Geometry: final body of the model. Coordinates: model frame, mm. A direction names the side the tool comes from. Coordinates: 2 decimals unless noted, no trailing zeros. Loops run counter-clockwise (first coordinate to the right, second up) from the corner with the lowest first, then second, coordinate; pieces in that order, holes last. Notation, with made-up numbers: (17.5, 7.5) -> (36.5, 7.5) arc R29 ccw to (36.5, 38.5) -> close; hole circle Ø2 at (89, 39). An arc over 180 degrees is marked (long way). One line per item, written item: value. Start each with the question number.
Item 1: Ray query, probe 1 along X at (y, z) = (60, 21); probe 2 along Y at (x, z) = (37.5, 12); probe 3 along Z at (x, y) = (37, -56.5). Return the intervals inside material, ascending. Write a range as from..to.
Item 2: Set-up query: faces 1 (the flat face through (1, 60, 30)), 2 (the cylindrical face through (39.81, 59.04, 14.79)), 3 (the flat face through (1, -41, 25)). Return all of +Z, -Z, +X, -X, +Y, -Y with unobstructed straight access to the full face (end or side cutting, diameter ignored); none if empty.
Item 3: Contact query for flat-ended pins moving along their axis: pin 1 Ø4 at (x, y) = (-37.5, 60) entering from +Z; pin 2 Ø2 at (x, y) = (26.5, 43.5) entering from -Z; pin 3 Ø4 at (x, y) = (22.5, -21) entering from +Z; pin 4 Ø3 at (x, y) = (-14, 59.5) entering from +Z. Output: stop coordinate, or through.
Item 4: Section query D-D on z = 32.5. Return loops of the section in (x, y).
Item 5: Section query A-A on y = -60. Return loops of the section in (x, z).
Item 6: Mould query, pull axis X, two halves, no side actions, for faces 4 (the flat face through (42.5, -1, 15)), 5 (the cylindrical face through (-36, -58, 12)), 6 (the flat face through (1, -7, 33)). Classes: +X half, -X half, draft (parallel to the pull), parting line (faces both ways), or undercut.
Item 7: Section query C-C on x = -25. Return loops of the section in (y, z).
Item 8: Section query B-B on x = -37.5. Return loops of the section in (y, z), then the cut area to 3 significant figures.
from build123d import *

# Parameters (mm, degrees)
SCHIZZO1_W                   = 85
SCHIZZO1_H                   = 130
SCHIZZO1_R                   = 2.5
ESTRUSIONE_ESTRUSIONE1_DEPTH = 40
TAGLIO_ESTRUSIONE1_DEPTH     = 115.236596588


with BuildPart() as part:
    # Schizzo1 → Estrusione-Estrusione1 (new body)
    with BuildSketch(Plane.XY):
        Rectangle(SCHIZZO1_W, SCHIZZO1_H)
        with Locations((-37.5, 60)):
            Circle(SCHIZZO1_R, mode=Mode.SUBTRACT)
        with Locations((37.5, 60)):
            Circle(SCHIZZO1_R, mode=Mode.SUBTRACT)
        with Locations((37.5, -60)):
            Circle(SCHIZZO1_R, mode=Mode.SUBTRACT)
        with Locations((-37.5, -60)):
            Circle(SCHIZZO1_R, mode=Mode.SUBTRACT)
    extrude(amount=ESTRUSIONE_ESTRUSIONE1_DEPTH)

    # Schizzo2 → Taglio-Estrusione1 (cut, through all)
    with BuildSketch(Plane(origin=(42.5, 0, 0), x_dir=(0, 0, -1), z_dir=(1, 0, 0))):
        Polygon((-40, 65), (-30, 65), (-30, 55), (-40, 45), align=None)
        with BuildLine():
            Line((-40, 0), (-40, -65))
            Line((-40, -65), (-25, -65))
            Line((-25, -65), (-25, -17.071067812))
            ThreePointArc((-25, -17.071067812), (-25.380602337, -15.15765065), (-26.464466094, -13.535533906))
            Line((-26.464466094, -13.535533906), (-40, 0))
        make_face()
    extrude(amount=-TAGLIO_ESTRUSIONE1_DEPTH, mode=Mode.SUBTRACT)


solid = part.part
Reply:
1. probe 1: x = -42.5..-40, -35..35, 40..42.5
1. probe 2: y = -65..-62.5, -57.5..57.5, 62.5..65
1. probe 3: z = 0..25
2. face 1: +Z, +X, -X, +Y
2. face 2: +Z, -Z
2. face 3: +Z, +X, -X, -Y
3. pin 1: passes through
3. pin 2: stops at z = 0
3. pin 3: stops at z = 25
3. pin 4: stops at z = 30
4. outline: (-42.5, -7.5) -> (42.5, -7.5) -> (42.5, 52.5) -> (-42.5, 52.5) -> close
5. outline: (-42.5, 0) -> (-40, 0) -> (-40, 25) -> (-42.5, 25) -> close; (-35, 0) -> (35, 0) -> (35, 25) -> (-35, 25) -> close; (40, 0) -> (42.5, 0) -> (42.5, 25) -> (40, 25) -> close
6. face 4: +X half
6. face 5: undercut
6. face 6: draft
7. outline: (-65, 0) -> (65, 0) -> (65, 30) -> (55, 30) -> (45, 40) -> (0, 40) -> (-13.54, 26.46) arc R5 cw to (-17.07, 25) -> (-65, 25) -> close
8. outline: (-65, 0) -> (-62.5, 0) -> (-62.5, 25) -> (-65, 25) -> close; (-57.5, 0) -> (57.5, 0) -> (57.5, 30) -> (55, 30) -> (45, 40) -> (0, 40) -> (-13.54, 26.46) arc R5 cw to (-17.07, 25) -> (-57.5, 25) -> close; (62.5, 0) -> (65, 0) -> (65, 30) -> (62.5, 30) -> close
8. area: 3,910 mm²
